Geometry: final body of the model. Coordinates: model frame, mm. Round coordinates to 2 decimals unless told otherwise and drop trailing zeros. Loops run counter-clockwise (first coordinate to the right, second up) from the corner with the lowest first, then second, coordinate; pieces in that order, holes last. Notation, with made-up numbers: M 25.25,23.5 L 45.25,23.5 A14 cw 45.25,41.5 Z; hole C 4.25,-15.75 d3. An arc over 180 degrees is marked long. Answer as a JSON object with one key per item and string values.
```python
from build123d import *

# Parameters (mm, degrees)
SKIZZE2_W                       = 240
SKIZZE2_H                       = 120
SKIZZE2_W_2                     = 10
SKIZZE2_H_2                     = 20
SKIZZE2_W_3                     = 20
SKIZZE2_H_3                     = 5
AUFSATZ_LINEAR_AUSTRAGEN1_DEPTH = 5
SKIZZE3_R                       = 2
SKIZZE3_R_2                     = 1.5
SCHNITT_LINEAR_AUSTRAGEN1_DEPTH = 146.430395722
SKIZZE4_R                       = 2
SCHNITT_LINEAR_AUSTRAGEN2_DEPTH = 146.430395722
SKIZZE6_W                       = 50
SKIZZE6_H                       = 67.054263566
SKIZZE6_W_2                     = 125.5
SKIZZE6_H_2                     = 20
SKIZZE6_W_3                     = 19.924
SKIZZE6_H_3                     = 55
SCHNITT_LINEAR_AUSTRAGEN3_DEPTH = 146.430395722


with BuildPart() as part:
    # Skizze2 → Aufsatz-Linear austragen1 (new body)
    with BuildSketch(Plane(origin=(0, 0, 0), x_dir=(0, 0, -1), z_dir=(1, 0, 0))):
        Rectangle(SKIZZE2_W, SKIZZE2_H)
        with Locations((-125, 50)):
            Rectangle(SKIZZE2_W_2, SKIZZE2_H_2)
        with Locations((125, 50)):
            Rectangle(SKIZZE2_W_2, SKIZZE2_H_2)
        with Locations((-90, -62.5)):
            Rectangle(SKIZZE2_W_3, SKIZZE2_H_3)
        with Locations((90, -62.5)):
            Rectangle(SKIZZE2_W_3, SKIZZE2_H_3)
    extrude(amount=AUFSATZ_LINEAR_AUSTRAGEN1_DEPTH)

    # Skizze3 → Schnitt-Linear austragen1 (cut, through all)
    with BuildSketch(Plane.ZY):
        with Locations((35.5, 46.5)):
            Circle(SKIZZE3_R)
        with Locations((100, 46.5)):
            Circle(SKIZZE3_R)
        with Locations((100, -40)):
            Circle(SKIZZE3_R)
        with Locations((35.5, -40)):
            Circle(SKIZZE3_R)
        with Locations((20.5, 31.5)):
            Circle(SKIZZE3_R_2)
        with Locations((-13.5, 31.5)):
            Circle(SKIZZE3_R_2)
        with Locations((-13.5, 16.5)):
            Circle(SKIZZE3_R_2)
        with Locations((20.5, 16.5)):
            Circle(SKIZZE3_R_2)
        with Locations((15.5, 1.5)):
            Circle(SKIZZE3_R_2)
        with Locations((15.5, -12)):
            Circle(SKIZZE3_R_2)
        with Locations((-8.5, 1.5)):
            Circle(SKIZZE3_R_2)
        with Locations((-8.5, -12)):
            Circle(SKIZZE3_R_2)
    extrude(amount=-SCHNITT_LINEAR_AUSTRAGEN1_DEPTH, mode=Mode.SUBTRACT)

    # Skizze4 → Schnitt-Linear austragen2 (cut, through all)
    with BuildSketch(Plane(origin=(5, 0, 0), x_dir=(0, 0, -1), z_dir=(1, 0, 0))):
        with Locations((63.424, 42.46)):
            Circle(SKIZZE4_R)
        with Locations((93.396, 26.46)):
            Circle(SKIZZE4_R)
        with Locations((63.424, 6.38)):
            Circle(SKIZZE4_R)
        with Locations((93.396, -9.62)):
            Circle(SKIZZE4_R)
    extrude(amount=-SCHNITT_LINEAR_AUSTRAGEN2_DEPTH, mode=Mode.SUBTRACT)

    # Skizze6 → Schnitt-Linear austragen3 (cut, through all)
    with BuildSketch(Plane(origin=(5, 0, 0), x_dir=(0, 0, -1), z_dir=(1, 0, 0))):
        with Locations((-67.75, 3.25)):
            Rectangle(SKIZZE6_W, SKIZZE6_H)
        with Locations((42.25, -35)):
            Rectangle(SKIZZE6_W_2, SKIZZE6_H_2)
        with Locations((38.462, 17.5)):
            Rectangle(SKIZZE6_W_3, SKIZZE6_H_3)
    extrude(amount=-SCHNITT_LINEAR_AUSTRAGEN3_DEPTH, mode=Mode.SUBTRACT)


solid = part.part
```
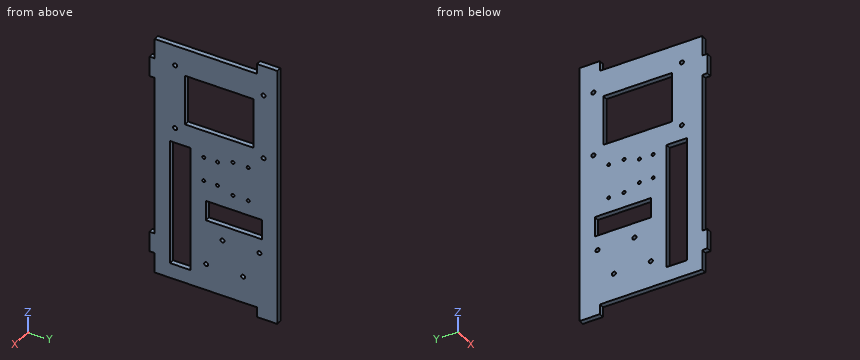
1) Cut plane B-B on z = 73. Return the cut outline in (x, y).
Geometry results:
{"outline": "M 0,-60 L 5,-60 L 5,-30.28 L 0,-30.28 Z; M 0,36.78 L 5,36.78 L 5,60 L 0,60 Z"}
2) Cut plane C-C on x = 3.2. Count the separate pieces of the cut face and the enclosed holes in it, and give its area (3 significant figures).
Geometry results:
{"separate pieces": "1", "enclosed holes": "19", "area": "22,300 mm2"}
3) Line query: probe 1 along Y at (x, z) = (2.5, -8.5); probe 2 along Y at (x, z) = (4.45, -42); probe 3 along Z at (x, y) = (2.35, -37). Output: solid intervals per line, ascending.
Geometry results:
{"probe 1": "-60 to -45, -25 to -13.5, -10.5 to 0, 3 to 60", "probe 2": "-60 to -45, -25 to -10, 45 to 60", "probe 3": "-120 to -105, 20.5 to 120"}
4) Cut plane A-A on z = -83. Return the cut outline in (x, y).
Geometry results:
{"outline": "M 0,-65 L 5,-65 L 5,-45 L 0,-45 Z; M 0,-25 L 5,-25 L 5,60 L 0,60 Z"}
5) First-contact query: pin 1 (2.5 mm diameter, centred on x = 3.5, y = -63, fed in from -Z); pin 2 (2.5 mm diameter, centred on x = 2.5, y = -63, fed in from +Z); pin 3 (3 mm diameter, centred on x = 2, z = 11.5, fed in from -Y). Flat tips, straight axial feed; report the tip coordinate or a pass-through.
Geometry results:
{"pin 1": "z = -100", "pin 2": "z = 100", "pin 3": "y = -60"}
